Part model, mm, in its own coordinate system. A direction names the side the tool comes from. Coordinates: 2 decimals unless noted, no trailing zeros. Loops run counter-clockwise (first coordinate to the right, second up) from the corner with the lowest first, then second, coordinate; pieces in that order, holes last.
```python
from build123d import *

# Parameters (mm, degrees)
BOSS_EXTRUDE1_DEPTH = 76.2
SKETCH4_W           = 12.7
SKETCH4_H           = 5.4864
CUT_EXTRUDE1_DEPTH  = 81.368682621
LPATTERN1_COUNT     = 6
LPATTERN1_PITCH     = 25.4
SKETCH5_R           = 2.5019
CUT_EXTRUDE2_DEPTH  = 81.435122899


with BuildPart() as part:
    # Sketch3 → Boss-Extrude1 (new, symmetric)
    with BuildSketch(Plane(origin=(0, 0, 0), x_dir=(0, 0, -1), z_dir=(1, 0, 0))):
        with BuildLine():
            Line((0, -2.7432), (-25.4, -2.7432))
            Line((-25.4, -2.7432), (-25.4, -1.524))
            Line((-25.4, -1.524), (0, -1.524))
            ThreePointArc((0, -1.524), (0.77286266, 1.313491267), (-1.332215689, -0.740119827))
            Line((-1.332215689, -0.740119827), (-2.39798824, -1.332215689))
            ThreePointArc((-2.39798824, -1.332215689), (1.391152789, 2.36428428), (0, -2.7432))
        make_face()
    extrude(amount=BOSS_EXTRUDE1_DEPTH, both=True)

    # Sketch4 → Cut-Extrude1 (cut, symmetric)
    with BuildSketch(Plane(origin=(0, 0, 0), x_dir=(1, 0, 0), z_dir=(0, 1, 0))):
        with Locations((-57.15, 0)):
            Rectangle(SKETCH4_W, SKETCH4_H)
    cut_extrude1 = extrude(amount=CUT_EXTRUDE1_DEPTH, both=True, mode=Mode.SUBTRACT)

    # LPattern1: Cut-Extrude1 ×6
    with Locations(*[(i * LPATTERN1_PITCH, 0, 0) for i in range(1, LPATTERN1_COUNT)]):
        add(cut_extrude1, mode=Mode.SUBTRACT)

    # Sketch5 → Cut-Extrude2 (cut, through all)
    with BuildSketch(Plane(origin=(0, -1.524, 0), x_dir=(1, 0, 0), z_dir=(0, 1, 0))):
        with Locations(Location((57.15, -14.224, 0), (0, 0, 270))):
            Circle(SKETCH5_R)
        with Locations(Location((-6.35, -14.224, 0), (0, 0, 270))):
            Circle(SKETCH5_R)
        with Locations(Location((-69.85, -14.224, 0), (0, 0, 270))):
            Circle(SKETCH5_R)
    extrude(amount=-CUT_EXTRUDE2_DEPTH, mode=Mode.SUBTRACT)


solid = part.part
```
Q1. Saw through at A-A (x = 57.15). List the corners of the cut face in (y, z), plus the area to 3 significant figures.
Q2. Mould opens along Z. For faces 4 (the cylindrical face through (31.839, 2.414, -1.304)), 5 (the cylindrical face through (-71, -2, 12)), 6 (the flat face through (0, -1.2, -1.2)) say: released by +Z, released by -Z, zero draft, split by the parting line, or undercut.
Q3. Drop flat-ended pins along their axis: P1, Ø10, axis at x = 19.5, z = 9, coming from the +Y side; P2, Ø2.5, axis at y = 1, z = -1, coming from the +X side. Give the stop position or say it passes through.
Q4. Tool access for faces 1 (the flat face through (63.5, -1.2, -1.2)), 2 (the cylindrical face through (6.439, 1.284, -0.82)), 3 (the flat face through (-12.7, -1.2, -1.2)): list every direction of +Z, -Z, +X, -X, +Y, -Y with a clear straight run to the whole face (end or side of a thin tool).
Q5. Probe line 1 (X direction, y = 1.1, z = 1.75); line 2 (Y direction, x = 32.5, z = 0). List the from-to ranges inside material, lowest first.
Q6. Saw through at B-B (x = 31). List the corners of the cut face in (y, z), plus the area to 3 significant figures.
Q7. Saw through at C-C (z = 22.5). List the corners of the cut face in (x, y).
Q8. Saw through at D-D (y = 0.55). Count the separate pieces of the cut face and the enclosed holes in it, plus the area to 3 significant figures.
Checked values:
1. outline: (-2.74, 0) arc R2.74 ccw (long way) to (-1.33, 2.4) - (-0.74, 1.33) arc R1.52 cw (long way) to (-1.52, 0) - (-1.52, 11.72) - (-2.74, 11.72) - close; (-2.74, 16.73) - (-1.52, 16.73) - (-1.52, 25.4) - (-2.74, 25.4) - close
1. area: 38.4 mm2
2. face 4: split by the parting line
2. face 5: undercut
2. face 6: zero draft
3. P1: stops at y = -1.52
3. P2: stops at x = 63.5
4. face 1: -Z, +X, +Y, -Y
4. face 2: +X, -X
4. face 3: -Z, +Y, -Y
5. line 1: x = -76.2 to -63.5, -50.8 to -38.1, -25.4 to -12.7, 0 to 12.7, 25.4 to 38.1, 50.8 to 63.5
5. line 2: y = -2.74 to -1.52, 1.52 to 2.74
6. outline: (-2.74, 0) arc R2.74 ccw (long way) to (-1.33, 2.4) - (-0.74, 1.33) arc R1.52 cw (long way) to (-1.52, 0) - (-1.52, 25.4) - (-2.74, 25.4) - close
6. area: 44.5 mm2
7. outline: (-76.2, -2.74) - (76.2, -2.74) - (76.2, -1.52) - (-76.2, -1.52) - close
8. separate pieces: 12
8. enclosed holes: 0
8. area: 193 mm2
